The model under review builds one solid part; all positions refer to its coordinate system, in mm. Coordinates: 2 decimals unless noted, no trailing zeros. Loops run counter-clockwise (first coordinate to the right, second up) from the corner with the lowest first, then second, coordinate; pieces in that order, holes last. Notation, with made-up numbers: (64, -1.5) - (117, -1.5) arc R15 cw to (117, 24.5) - close; hole circle Ø2 at (64.25, 45.25). An arc over 180 degrees is marked (long way). One line per item, written item: value. Start each with the question number.
1. We need section C-C, the plane z = 3.75. Give the boundary of the cut face in (x, y).
2. To check wall thickness, follow line 1 (Z direction, x = 8, y = -15.5); line 2 (X direction, y = -46, z = 4.5); line 3 (Y direction, x = 0, z = 6.3). State the ranges of each line that lie inside material, in increasing order.
3. Insertion check: P1, Ø3, axis at x = -12, z = 2, coming from the -Y side; P2, Ø1, axis at x = -16, z = 1.5, coming from the -Y side; P3, Ø4, axis at x = 18.5, y = 52, coming from the +Z side. Each pin has a flat end and moves straight along its axis. Give the tip position at first contact, or say it passes through.
4. Mouldability with a two-part tool opening along X and no side actions: class faces 1 (the face through (-1, 1, 2.54)), 2 (the face through (-1, 1, 0)) as +X half, -X half, draft (parallel to the pull), parting line (faces both ways), or undercut.
from build123d import *

# Parameters (mm, degrees)
F0_R     = 69.85
F1_DEPTH = 6.35
F2_R     = 6.34999
F3_T     = 2.54


# Not quite as in the source:
# - a fillet or chamfer is up to 0.001 mm smaller than in the source, because OpenCascade refuses the exact size
# - a shell that OpenCascade refuses in one call is made with other operations: the cavity is built on its own and cut out


with BuildPart() as f1:
    # F0 (on Top) → F1 (new body)
    with BuildSketch(Plane.XY):
        Circle(F0_R)
    extrude(amount=F1_DEPTH)

    # F2 (radius 6.35 in the source; OpenCascade refuses exactly that, so slightly less here)
    f2_edges = [f1.edges().sort_by_distance(p)[0] for p in [
        (-69.85, 0, 0),
    ]]
    fillet(f2_edges, radius=F2_R)

    # F3: shell of thickness 2.54, made by hand


with BuildPart() as f3_core1:
    # F3_t2: copy of F1
    add(f1.part)

    # the walls: a layer under each face that stays
    f3_faces = [f3_core1.faces().sort_by_distance(p)[0] for p in [
        (-69.85, 0, 6.349995),
        (-67.9901309895, 0, 1.8598690105),
        (0, 0, 0),
    ]]
    thicken(f3_faces, amount=-F3_T, mode=Mode.SUBTRACT)


with BuildPart() as f1_1:
    add(f1.part)

    # what is left inside the walls is the cavity
    f3_cavity = [f3_core1.part.solids().sort_by_distance(p)[0] for p in [
        (0, -22.436667, 6.3246),
    ]]
    add(f3_cavity, mode=Mode.SUBTRACT)


solid = f1_1.part
Findings below:
1. outline: circle Ø138.59 at (0, 0); hole circle Ø132.57 at (0, 0)
2. line 1: 0 to 2.54
2. line 2: -52.2 to -48.48, 48.48 to 52.2
2. line 3: -69.85 to -67.31, 67.31 to 69.85
3. P1: y = -68.17
3. P2: y = -66.24
3. P3: z = 2.54
4. face 1: undercut
4. face 2: draft
